Model file for the job. Use its own axes, mm. A direction names the side the tool comes from. Coordinates: 2 decimals unless noted, no trailing zeros. Write each loop counter-clockwise with the first axis right and the second up, starting at its lowest first coordinate (ties: lowest second). Pieces come first, ordered by that corner, then holes. Notation, with made-up numbers: (16.5, 69) -> (67.5, 69) arc R17 cw to (67.5, 81) -> close; hole circle Ø11 at (34.5, 47.25). An arc over 180 degrees is marked (long way). Answer as a JSON object with one key per item and string values. Group by question number.
from build123d import *

# Parameters (mm, degrees)
BOSS_EXTRUDE1_DEPTH      = 4.5
BOSS_EXTRUDE1_DEPTH_BACK = 4.5
CUT_EXTRUDE1_DEPTH       = 2.1
CUT_EXTRUDE1_DEPTH_BACK  = 2.1
BOSS_EXTRUDE2_DEPTH      = 3
BOSS_EXTRUDE2_DEPTH_BACK = 3
SKETCH2_W                = 6
SKETCH2_H                = 6
SKETCH2_R                = 1.25
FILLET2_R                = 1.5
SKETCH5_W                = 120
SKETCH5_H                = 30
CUT_EXTRUDE2_DEPTH       = 68.825142831


with BuildPart() as part:
    # Sketch1 → Boss-Extrude1 (new, two sides: drawn at the far end of the back side and taken through both)
    # profile 1 of 2: a face of its own
    with BuildSketch(Plane(origin=(0, 0, 0), x_dir=(1, 0, 0), z_dir=(0, 1, 0)).offset(-BOSS_EXTRUDE1_DEPTH_BACK)):
        with BuildLine():
            Line((-24, 50), (24, 50))
            ThreePointArc((24, 50), (33.899494937, 45.899494937), (38, 36))
            Line((38, 36), (38, 20.869079534))
            Line((38, 20.869079534), (35.573892834, -34.697910198))
            ThreePointArc((35.573892834, -34.697910198), (30.653330181, -45.557823393), (19.589121288, -50))
            Line((19.589121288, -50), (-19.589121288, -50))
            ThreePointArc((-19.589121288, -50), (-30.653330181, -45.557823393), (-35.573892834, -34.697910198))
            Line((-35.573892834, -34.697910198), (-38, 20.869079534))
            Line((-38, 20.869079534), (-38, 36))
            ThreePointArc((-38, 36), (-33.899494937, 45.899494937), (-24, 50))
        make_face()
        with BuildLine():
            ThreePointArc((-24, 46.7), (-31.566042559, 43.566042559), (-34.7, 36))
            Line((-34.7, 36), (-34.7, 20.94108579))
            Line((-34.7, 20.94108579), (-32.277033702, -34.55396622))
            ThreePointArc((-32.277033702, -34.55396622), (-28.371337097, -43.174022318), (-19.589121288, -46.7))
            Line((-19.589121288, -46.7), (19.589121288, -46.7))
            ThreePointArc((19.589121288, -46.7), (28.371337097, -43.174022318), (32.277033702, -34.55396622))
            Line((32.277033702, -34.55396622), (34.7, 20.94108579))
            Line((34.7, 20.94108579), (34.7, 36))
            ThreePointArc((34.7, 36), (31.566042559, 43.566042559), (24, 46.7))
            Line((24, 46.7), (-24, 46.7))
        make_face(mode=Mode.SUBTRACT)
    # profile 2 of 2: a face of its own
    with BuildSketch(Plane(origin=(0, 0, 0), x_dir=(1, 0, 0), z_dir=(0, 1, 0)).offset(-BOSS_EXTRUDE1_DEPTH_BACK)):
        with BuildLine():
            Line((-24, 46.7), (24, 46.7))
            ThreePointArc((24, 46.7), (31.566042559, 43.566042559), (34.7, 36))
            Line((34.7, 36), (34.7, 20.94108579))
            Line((34.7, 20.94108579), (32.277033702, -34.55396622))
            ThreePointArc((32.277033702, -34.55396622), (28.371337097, -43.174022318), (19.589121288, -46.7))
            Line((19.589121288, -46.7), (-19.589121288, -46.7))
            ThreePointArc((-19.589121288, -46.7), (-28.371337097, -43.174022318), (-32.277033702, -34.55396622))
            Line((-32.277033702, -34.55396622), (-34.7, 20.94108579))
            Line((-34.7, 20.94108579), (-34.7, 36))
            ThreePointArc((-34.7, 36), (-31.566042559, 43.566042559), (-24, 46.7))
        make_face()
        with BuildLine():
            ThreePointArc((-24, 44.6), (-30.081118318, 42.081118318), (-32.6, 36))
            Line((-32.6, 36), (-32.6, 20.986907953))
            Line((-32.6, 20.986907953), (-30.179032437, -34.462365506))
            ThreePointArc((-30.179032437, -34.462365506), (-26.91915968, -41.657057998), (-19.589121288, -44.6))
            Line((-19.589121288, -44.6), (19.589121288, -44.6))
            ThreePointArc((19.589121288, -44.6), (26.91915968, -41.657057998), (30.179032437, -34.462365506))
            Line((30.179032437, -34.462365506), (32.6, 20.986907953))
            Line((32.6, 20.986907953), (32.6, 36))
            ThreePointArc((32.6, 36), (30.081118318, 42.081118318), (24, 44.6))
            Line((24, 44.6), (-24, 44.6))
        make_face(mode=Mode.SUBTRACT)
    extrude(amount=BOSS_EXTRUDE1_DEPTH + BOSS_EXTRUDE1_DEPTH_BACK)

    # Sketch1<3> → Cut-Extrude1 (cut, two sides: drawn at the far end of the back side and taken through both)
    with BuildSketch(Plane(origin=(0, 0, 0), x_dir=(1, 0, 0), z_dir=(0, 1, 0)).offset(-CUT_EXTRUDE1_DEPTH_BACK)):
        with BuildLine():
            Line((-24, 46.7), (24, 46.7))
            ThreePointArc((24, 46.7), (31.566042559, 43.566042559), (34.7, 36))
            Line((34.7, 36), (34.7, 20.94108579))
            Line((34.7, 20.94108579), (32.277033702, -34.55396622))
            ThreePointArc((32.277033702, -34.55396622), (28.371337097, -43.174022318), (19.589121288, -46.7))
            Line((19.589121288, -46.7), (-19.589121288, -46.7))
            ThreePointArc((-19.589121288, -46.7), (-28.371337097, -43.174022318), (-32.277033702, -34.55396622))
            Line((-32.277033702, -34.55396622), (-34.7, 20.94108579))
            Line((-34.7, 20.94108579), (-34.7, 36))
            ThreePointArc((-34.7, 36), (-31.566042559, 43.566042559), (-24, 46.7))
        make_face()
        with BuildLine():
            Line((-32, 36), (-32, 21))
            Line((-32, 21), (-29.579603504, -34.436193874))
            ThreePointArc((-29.579603504, -34.436193874), (-26.504251846, -41.223639621), (-19.589121288, -44))
            Line((-19.589121288, -44), (19.589121288, -44))
            ThreePointArc((19.589121288, -44), (26.504251846, -41.223639621), (29.579603504, -34.436193874))
            Line((29.579603504, -34.436193874), (32, 21))
            Line((32, 21), (32, 36))
            ThreePointArc((32, 36), (29.656854249, 41.656854249), (24, 44))
            Line((24, 44), (-24, 44))
            ThreePointArc((-24, 44), (-29.656854249, 41.656854249), (-32, 36))
        make_face(mode=Mode.SUBTRACT)
    extrude(amount=CUT_EXTRUDE1_DEPTH + CUT_EXTRUDE1_DEPTH_BACK, mode=Mode.SUBTRACT)

    # Sketch2 → Boss-Extrude2 (add, two sides: drawn at the far end of the back side and taken through both)
    # profile 1 of 2: a face of its own
    with BuildSketch(Plane(origin=(0, 0, 0), x_dir=(0, 0, -1), z_dir=(1, 0, 0)).offset(-BOSS_EXTRUDE2_DEPTH_BACK)):
        with Locations((-53, 0)):
            Rectangle(SKETCH2_W, SKETCH2_H)
        with Locations((-53, 0)):
            Circle(SKETCH2_R, mode=Mode.SUBTRACT)
    # profile 2 of 2: a face of its own
    with BuildSketch(Plane(origin=(0, 0, 0), x_dir=(0, 0, -1), z_dir=(1, 0, 0)).offset(-BOSS_EXTRUDE2_DEPTH_BACK)):
        with Locations((53, 0)):
            Rectangle(SKETCH2_W, SKETCH2_H)
        with Locations((53, 0)):
            Circle(SKETCH2_R, mode=Mode.SUBTRACT)
    extrude(amount=BOSS_EXTRUDE2_DEPTH + BOSS_EXTRUDE2_DEPTH_BACK)

    # Fillet2
    fillet2_edges = [part.edges().sort_by_distance(p)[0] for p in [
        (0, 3, 50),
        (0, -3, 50),
        (0, -3, -50),
        (0, 3, -50),
    ]]
    fillet(fillet2_edges, radius=FILLET2_R - 0.0001)  # a hair under: the kernel refuses the full size

    # Sketch5 → Cut-Extrude2 (cut, through all)
    with BuildSketch(Plane(origin=(0, 0, 0), x_dir=(0, 0, -1), z_dir=(1, 0, 0))):
        Rectangle(SKETCH5_W, SKETCH5_H)
    extrude(amount=-CUT_EXTRUDE2_DEPTH, mode=Mode.SUBTRACT)


solid = part.part
(1) 3-axis set-ups, long thin cutter, end or side, ignore diameter. For faces 5 (the face through (3, 0.1, -51.6)), 6 (the face through (26.84, -3.32, 41.73)), 7 (the face through (33, 2.1, -4)), 8 (the face through (1, -3, -54)), 9 (the face through (3, -1, 52)): which of +Z, -Z, +X, -X, +Y, -Y reach the whole face in a straight line?
(2) Cut at A-A on y = 0. List the corners of the cut face in (x, z), plus the area to 3 significant figures.
(3) Pull direction Y, two halves, no side cores. Call faces 1 (the face through (1, -3, 54)), 2 (the face through (31.48, -0.03, -43.65)), 3 (the face through (12, 0, -46.7)), 4 (the face through (30.15, -3.32, -42.01)): released by +Y, released by -Y, zero draft, split by the parting line, or undercut.
(4) Pin check, flat tips, straight feed: pin 1 (2 mm diameter, centred on y = 0.5, z = -26, fed in from -X); pin 2 (0.7 mm diameter, centred on x = 10.5, y = 3, fed in from -Z); pin 3 (1.2 mm diameter, centred on x = 10.5, y = 3, fed in from +Z). Stop position of each tip, or through.
(5) Cut at C-C on z = 53. List the corners of the cut face in (x, y), plus the area to 3 significant figures.
(6) Cut at B-B on x = 6.5. List the corners of the cut face in (y, z).
(7) Wall check: probe 1 along Z at (x, y) = (1.2, 0); probe 2 along Y at (x, z) = (2, 53); probe 3 along Z at (x, y) = (12, 3.75). Give the ranges that are in metal, low to high.
(8) Cut at D-D on z = 36.5. List the corners of the cut face in (x, y), plus the area to 3 significant figures.
Results found:
{
 "1": {"face 5": "-Z, +X, +Y, -Y", "face 6": "-X, +Y, -Y", "face 7": "-X", "face 8": "-Z, +X, -X, -Y", "face 9": "+Z, +X, +Y, -Y"},
 "2": {"outline": "(0, -56) -> (3, -56) -> (3, -54.25) -> (0, -54.25) -> close; (0, -51.75) -> (3, -51.75) -> (3, -50) -> (24, -50) arc R14 ccw to (38, -36) -> (38, -20.87) -> (35.57, 34.7) arc R16 ccw to (19.59, 50) -> (3, 50) -> (3, 51.75) -> (0, 51.75) -> (0, 46.7) -> (19.59, 46.7) arc R12.7 cw to (32.28, 34.55) -> (34.7, -20.94) -> (34.7, -36) arc R10.7 cw to (24, -46.7) -> (0, -46.7) -> close; (0, 54.25) -> (3, 54.25) -> (3, 56) -> (0, 56) -> close", "area": "534 mm²"},
 "3": {"face 1": "released by -Y", "face 2": "undercut", "face 3": "undercut", "face 4": "zero draft"},
 "4": {"pin 1": "stops at x = 34.7", "pin 2": "stops at z = -50", "pin 3": "stops at z = 50"},
 "5": {"outline": "(0, -3) -> (3, -3) -> (3, -1.25) -> (0, -1.25) -> close; (0, 1.25) -> (3, 1.25) -> (3, 3) -> (0, 3) -> close", "area": "10.5 mm²"},
 "6": {"outline": "(-4.5, -50) -> (4.5, -50) -> (4.5, -44.6) -> (2.1, -44.6) -> (2.1, -46.7) -> (-2.1, -46.7) -> (-2.1, -44.6) -> (-4.5, -44.6) -> close; (-4.5, 44.6) -> (-2.1, 44.6) -> (-2.1, 46.7) -> (2.1, 46.7) -> (2.1, 44.6) -> (4.5, 44.6) -> (4.5, 50) -> (-4.5, 50) -> close"},
 "7": {"probe 1": "z = -56 to -54.25, -51.75 to -46.7, 46.7 to 51.75, 54.25 to 56", "probe 2": "y = -3 to -1.25, 1.25 to 3", "probe 3": "z = -50 to -44.6, 44.6 to 50"},
 "8": {"outline": "(29.89, -4.5) -> (35.39, -4.5) -> (35.39, 4.5) -> (29.89, 4.5) -> (29.89, 2.1) -> (32.04, 2.1) -> (32.04, -2.1) -> (29.89, -2.1) -> close", "area": "40.5 mm²"}
}
